Design review of the part built by this model. Coordinates are the model's own, in mm. Face numbers are marked on the shaded views. A direction names the side the tool comes from. Round coordinates to 2 decimals unless told otherwise and drop trailing zeros. Write each loop counter-clockwise with the first axis right and the second up, starting at its lowest first coordinate (ties: lowest second). Pieces come first, ordered by that corner, then holes. Notation, with made-up numbers: (87, -7) -> (145, -7) arc R25 cw to (145, 16) -> close; hole circle Ø9 at (-1, 0.25). An arc over 180 degrees is marked (long way). One line per question, with ' | ' between items. Start each with the question number.
1) Consider section A-A (x = 0). Give the boundary of the cut face in (y, z).
2) Consider section D-D (z = 6). Give the boundary of the cut face in (x, y).
3) For probe 1 along Z at (x, y) = (2.5, 1.25); probe 2 along Y at (x, z) = (0, 1.9); probe 3 along X at (y, z) = (0, 1.5), list the stretches that pass through material, from the lowest coordinate up.
4) Consider section C-C (z = 1). Give the boundary of the cut face in (x, y).
5) Consider section B-B (y = 4.5). Give the boundary of the cut face in (x, z).
6) For the marked faces 4 and 5, list the 3-axis set-ups (+Z, -Z, +X, -X, +Y, -Y) from which the entire face can be reached by the end or side of a thin tool; tool diameter is ignored.
7) Mouldability with a two-part tool opening along Z and no side actions: class the marked faces 1, 2 and 3 as +Z half, -Z half, draft (parallel to the pull), parting line (faces both ways), or undercut.
8) Insertion check: pin 1 Ø1 at (x, z) = (-21.5, 6.5) entering from +Y; pin 2 Ø1.5 at (x, z) = (-17.5, 1.5) entering from -Y; pin 3 Ø1 at (y, z) = (2, 1.5) entering from +X; pin 4 Ø8 at (x, y) = (-14.5, 2.5) entering from -Z. Each pin has a flat end and moves straight along its axis. Give the tip position at first contact, or say it passes through.
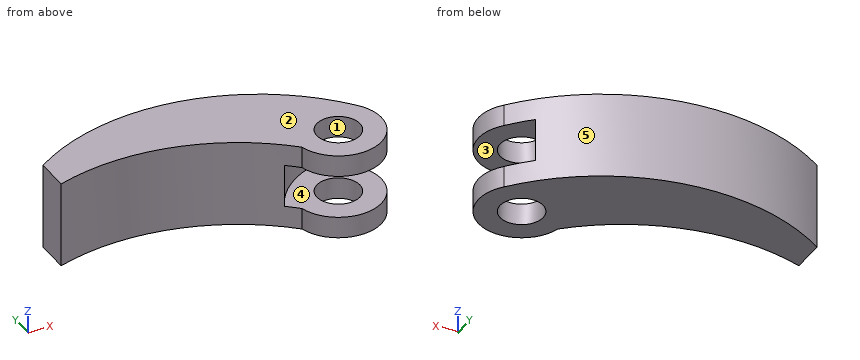
```python
from build123d import *

# Parameters (mm, degrees)
SKETCH1_R               = 5
BOSS_EXTRUDE1_DEPTH     = 10
SKETCH2_R               = 2.5
CUT_EXTRUDE1_DEPTH      = 13.247448714
BOSS_EXTRUDE2_DEPTH     = 10
SKETCH7_R               = 2.5
CUT_EXTRUDE2_DEPTH      = 35.052803759
CUT_EXTRUDE4_DEPTH      = 2.5
CUT_EXTRUDE4_DEPTH_BACK = 2.5
SKETCH15_R              = 10


with BuildPart() as part:
    # Sketch1 → Boss-Extrude1 (new body)
    with BuildSketch(Plane.XY):
        Circle(SKETCH1_R)
    extrude(amount=BOSS_EXTRUDE1_DEPTH)

    # Sketch2 → Cut-Extrude1 (cut, through all)
    with BuildSketch(Plane.XY.offset(10)):
        Circle(SKETCH2_R)
    extrude(amount=-CUT_EXTRUDE1_DEPTH, mode=Mode.SUBTRACT)

    # Sketch6 → Boss-Extrude2 (add)
    with BuildSketch(Plane.XY):
        with BuildLine():
            Line((-30, 8.156486671), (-30, 4.156486671))
            ThreePointArc((-30, 4.156486671), (-16.68023923, 4.957359729), (-4.845860122, -1.207451361))
            Line((-4.845860122, -1.207451361), (3.769015533, 3.285501775))
            ThreePointArc((3.769015533, 3.285501775), (-12.155410699, 12.376939364), (-30, 8.156486671))
        make_face()
    extrude(amount=BOSS_EXTRUDE2_DEPTH)

    # Sketch7 → Cut-Extrude2 (cut, through all)
    with BuildSketch(Plane.XY.offset(10)):
        Circle(SKETCH7_R)
    extrude(amount=-CUT_EXTRUDE2_DEPTH, mode=Mode.SUBTRACT)

    # Sketch15 → Cut-Extrude4 (cut, two sides: drawn at the far end of the back side and taken through both)
    with BuildSketch(Plane.XY.offset(5).offset(-CUT_EXTRUDE4_DEPTH_BACK)):
        with Locations((2.839216425, -4.115683429)):
            Circle(SKETCH15_R)
    extrude(amount=CUT_EXTRUDE4_DEPTH + CUT_EXTRUDE4_DEPTH_BACK, mode=Mode.SUBTRACT)


solid = part.part
```
From the geometry:
1) outline: (-5, 0) -> (-2.5, 0) -> (-2.5, 2.5) -> (-5, 2.5) -> close; (-5, 7.5) -> (-2.5, 7.5) -> (-2.5, 10) -> (-5, 10) -> close; (2.5, 0) -> (7.07, 0) -> (7.07, 10) -> (2.5, 10) -> (2.5, 7.5) -> (5.47, 7.5) -> (5.47, 2.5) -> (2.5, 2.5) -> close
2) outline: (-30, 4.16) arc R25 cw to (-6.27, 0.02) arc R10 cw to (1.46, 5.79) arc R25 ccw to (-30, 8.16) -> close
3) probe 1: z = 0 to 2.5, 7.5 to 10 | probe 2: y = -5 to -2.5, 2.5 to 7.07 | probe 3: x = -6.24 to -2.5, 2.5 to 5
4) outline: (-30, 4.16) arc R25 cw to (-4.85, -1.2) arc R5 ccw (long way) to (3.77, 3.29) arc R25 ccw to (-30, 8.16) -> close; hole circle Ø5 at (0, 0)
5) outline: (-30, 0) -> (-28.92, 0) -> (-28.92, 10) -> (-30, 10) -> close; (-14.87, 0) -> (2.73, 0) -> (2.73, 2.5) -> (-2.24, 2.5) -> (-2.24, 7.5) -> (2.73, 7.5) -> (2.73, 10) -> (-14.87, 10) -> close
6) face 4: +X, -Y | face 5: +Z, -Z, +Y
7) face 1: draft | face 2: +Z half | face 3: undercut
8) pin 1: stops at y = 12.07 | pin 2: stops at y = 4.97 | pin 3: stops at x = 4.77 | pin 4: stops at z = 0
